Here's how the part is built. I have some questions about the finished solid (model axes, mm). A direction names the side the tool comes from. Give positions to 0.01 mm unless a question says otherwise; leave off trailing zeros. Order: outer loops, then holes, each group sorted by start corner. A loop starts at its lowest first (then second) coordinate and runs counter-clockwise, first axis right, second up. Notation, with made-up numbers: (-0.5, -16) - (20.5, -16) arc R25 ccw to (20.5, 23) - close; hole circle Ø11 at (22.5, 21.25). An arc over 180 degrees is marked (long way). One line per question, with ' | ' between items.
from build123d import *

# Parameters (mm, degrees)
F0_R      = 19.75
F1_DEPTH  = 17
F2_R      = 18.25
F3_DEPTH  = 15
F4_R      = 9.5
F5_DEPTH  = 14.5
F6_R      = 9.25
F7_DEPTH  = 14
F8_R      = 3.2
F9_DEPTH  = 9.2
F10_R     = 1.6
F11_DEPTH = 7
F12_R     = 2.25
F13_DEPTH = 25.4
F14_R     = 3.5
F15_DEPTH = 2
F16_R     = 2
F17_DEPTH = 2
F18_R     = 0.4
F19_DEPTH = 0.5


with BuildPart() as f1:
    # F0 (on Front) → F1 (new body)
    with BuildSketch(Plane.XZ):
        Circle(F0_R)
    extrude(amount=F1_DEPTH)

    # F2 (on face) → F3 (cut)
    with BuildSketch(Plane.XZ.offset(17)):
        Circle(F2_R)
    extrude(amount=-F3_DEPTH, mode=Mode.SUBTRACT)

    # F4 (on face) → F5 (join)
    with BuildSketch(Plane(origin=(0, 0, 0), x_dir=(-1, 0, 0), z_dir=(0, 1, 0))):
        Circle(F4_R)
    extrude(amount=-F5_DEPTH)

    # F6 (on face) → F7 (cut)
    with BuildSketch(Plane(origin=(0, 0, 0), x_dir=(-1, 0, 0), z_dir=(0, 1, 0))):
        Circle(F6_R)
    extrude(amount=-F7_DEPTH, mode=Mode.SUBTRACT)

    # F8 (on face) → F9 (join)
    with BuildSketch(Plane.XZ.offset(14.5)):
        Circle(F8_R)
    extrude(amount=F9_DEPTH)

    # F10 (on face) → F11 (cut)
    with BuildSketch(Plane.XZ.offset(23.7)):
        Circle(F10_R)
    extrude(amount=-F11_DEPTH, mode=Mode.SUBTRACT)

    # F12 (on face) → F13 (cut)
    with BuildSketch(Plane.XZ.offset(14.5)):
        with Locations((-2.813868, 6.090039)):
            Circle(F12_R)
        with Locations((2.316602, 6.296013)):
            Circle(F12_R)
        with Locations((6.090039, 2.813868)):
            Circle(F12_R)
        with Locations((6.296013, -2.316602)):
            Circle(F12_R)
        with Locations((2.813868, -6.090039)):
            Circle(F12_R)
        with Locations((-2.316602, -6.296013)):
            Circle(F12_R)
        with Locations((-6.090039, -2.813868)):
            Circle(F12_R)
        with Locations((-6.296013, 2.316602)):
            Circle(F12_R)
    extrude(amount=-F13_DEPTH, mode=Mode.SUBTRACT)

    # F14 (on face) → F15 (join)
    with BuildSketch(Plane(origin=(0, -14, 0), x_dir=(-1, 0, 0), z_dir=(0, 1, 0))):
        Circle(F14_R)
    extrude(amount=F15_DEPTH)

    # F16 (on face) → F17 (join)
    with BuildSketch(Plane(origin=(0, -12, 0), x_dir=(-1, 0, 0), z_dir=(0, 1, 0))):
        Circle(F16_R)
    extrude(amount=F17_DEPTH)

    # F18 (on face) → F19 (join)
    with BuildSketch(Plane(origin=(0, -12, 0), x_dir=(-1, 0, 0), z_dir=(0, 1, 0))):
        with Locations((-2.139466, -1.804263)):
            Circle(F18_R)
        with Locations((-0.670345, -2.717225)):
            Circle(F18_R)
        with Locations((1.054824, -2.592301)):
            Circle(F18_R)
        with Locations((2.377087, -1.477205)):
            Circle(F18_R)
        with Locations((2.791383, 0.202133)):
            Circle(F18_R)
        with Locations((2.139466, 1.804263)):
            Circle(F18_R)
        with Locations((0.670345, 2.717225)):
            Circle(F18_R)
        with Locations((-1.054824, 2.592301)):
            Circle(F18_R)
        with Locations((-2.791383, -0.202133)):
            Circle(F18_R)
        with Locations((-2.377087, 1.477205)):
            Circle(F18_R)
    extrude(amount=F19_DEPTH)


solid = f1.part
1) Please list where these lines run through material, in increasing order: L1, parallel to Z at x = 0, y = -7.5; L2, parallel to X at y = -3.75, z = 1; L3, parallel to Z at x = 0, y = -18.75.
Model answer:
L1: z = -19.75 to -18.25, -9.5 to -9.25, 9.25 to 9.5, 18.25 to 19.75 | L2: x = -19.72 to -18.22, -9.45 to -9.2, 9.2 to 9.45, 18.22 to 19.72 | L3: z = -3.2 to -1.6, 1.6 to 3.2
2) Thinking about a two-plate mould opening in X: for faces 1 (the face through (17.5, -17, -5.8)), 2 (the face through (-1.27, -20.25, -0.97)), which applies, +X half, -X half, draft (parallel to the pull), parting line (faces both ways), or undercut?
Model answer:
face 1: draft | face 2: undercut
3) I want a section at B-B (z = 7). List the corners of the cut face in (x, y) for me, plus the area to 3 significant figures.
Model answer:
outline: (-18.47, -17) - (-16.85, -17) - (-16.85, -2) - (-6.42, -2) - (-6.42, -14.5) - (-4.87, -14.5) - (-4.87, -14) - (-6.05, -14) - (-6.05, 0) - (-18.47, 0) - close; (-0.76, -14.5) - (0.18, -14.5) - (0.18, -14) - (-0.76, -14) - close; (4.45, -14.5) - (6.42, -14.5) - (6.42, -2) - (16.85, -2) - (16.85, -17) - (18.47, -17) - (18.47, 0) - (6.05, 0) - (6.05, -14) - (4.45, -14) - close | area: 109 mm2
4) On a 3-axis mill with a long thin cutter (end or side, diameter ignored), from which of +Z, -Z, +X, -X, +Y, -Y can I reach the whole of each face in a straight line? I mean faces 3 (the face through (-1.78, -14.25, 4.09)), 4 (the face through (-2, -12, -2)), 5 (the face through (8, -2, -8)). Say none if no direction works.
Model answer:
face 3: +Y, -Y | face 4: +Y | face 5: -Y
5) I want a section at D-D (y = -20.5). List the corners of the cut face in (x, z) for me.
Model answer:
outline: circle Ø6.4 at (0, 0); hole circle Ø3.2 at (0, 0)
6) I'm going to push flat-ended pins straight in: P1, Ø5, axis at y = -10, z = 12, coming from the +X side; P2, Ø2, axis at x = -5, y = -15, coming from the +Z side; P3, Ø12, axis at x = -6.5, z = -7, coming from the -Y side; P4, Ø5, axis at y = -20.5, z = -8, coming from the -X side. Where does each tip first touch, or does it pass through?
Model answer:
P1: stops at x = 17.32 | P2: stops at z = 19.34 | P3: stops at y = -14.5 | P4: passes through
7) I want a section at A-A (y = -4.5). List the corners of the cut face in (x, z) for me.
Model answer:
outline: circle Ø39.5 at (0, 0); circle Ø19 at (0, 0); hole circle Ø36.5 at (0, 0); hole circle Ø18.5 at (0, 0)
8) I want a section at C-C (x = 16). List the corners of the cut face in (y, z) for me.
Model answer:
outline: (-17, -11.58) - (0, -11.58) - (0, 11.58) - (-17, 11.58) - (-17, 8.78) - (-2, 8.78) - (-2, -8.78) - (-17, -8.78) - close
